Could you check a few things on this model? Use its own coordinates, in mm. Face numbers are marked on the shaded views. Round coordinates to 2 decimals unless told otherwise and drop trailing zeros. Loops run counter-clockwise (first coordinate to the right, second up) from the corner with the lowest first, then second, coordinate; pieces in that order, holes last. Notation, with made-up numbers: M 57,-13.5 L 115,-13.5 A14 ccw 115,13.5 Z; hole C 81.5,12.5 d7. An arc over 180 degrees is marked long. Answer in a Markdown table with one row per item.
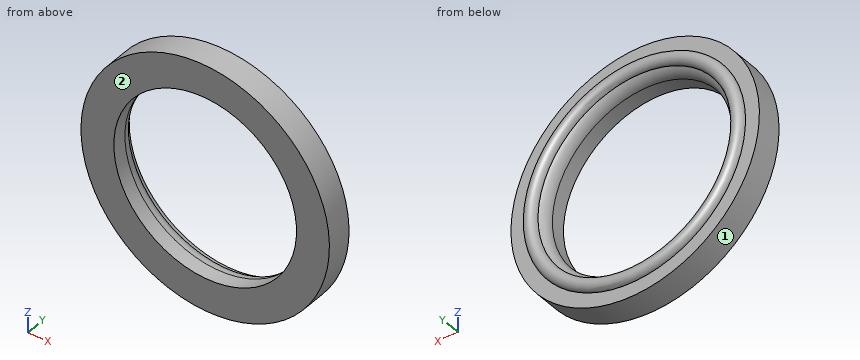
```python
from build123d import *

# Parameters (mm, degrees)
SKETCH1_R           = 23.0505
SKETCH1_R_2         = 16.9545
BOSS_EXTRUDE1_DEPTH = 4.7625
FILLET1_R           = 2.54


with BuildPart() as part:
    # Sketch1 → Boss-Extrude1 (new body)
    with BuildSketch(Plane(origin=(0, 0, 0), x_dir=(1, 0, 0), z_dir=(0, 1, 0))):
        with Locations(Location((0, 0, 0), (0, 0, 90))):
            Circle(SKETCH1_R)
        with Locations(Location((0, 0, 0), (0, 0, 90))):
            Circle(SKETCH1_R_2, mode=Mode.SUBTRACT)
    extrude(amount=BOSS_EXTRUDE1_DEPTH)

    # Sketch2 → Revolve1 (revolve)
    with BuildSketch(Plane.XY, mode=Mode.PRIVATE) as revolve1_sk:
        with BuildLine():
            Line((18.034, 4.710412046), (20.477314517, 4.739986951))
            ThreePointArc((20.477314517, 4.739986951), (19.240869806, 5.946856757), (18.034, 4.710412046))
        make_face()
    revolve(revolve1_sk.sketch.rotate(Axis((0, 0, 0), (0, 1, 0)), 90), axis=Axis((0, 0, 0), (0, 1, 0)))

    # Fillet1
    # the kernel refuses this fillet: 2.54 mm, written as the material it takes off along each edge
    with BuildSketch(Plane(origin=(0, 4.7625, 0), x_dir=(0, 0, -1), z_dir=(1, 0, 0))) as fillet1_piece_1:
        with BuildLine():
            CenterArc((19.4945, -2.078446948), FILLET1_R, 125.086398031, 54.913601969)
            Line((18.03448004, 0), (18.005279641, 0.041568939))
            ThreePointArc((18.005279641, 0.041568939), (17.49449002, 0.0508), (16.9545, 0.0508))
            Line((16.9545, 0.0508), (16.9037, 0))
            Line((16.9037, 0), (16.9037, -2.078446948))
            Line((16.9037, -2.078446948), (16.9545, -2.078446948))
        make_face()
    revolve(axis=Axis((0, 4.7625, 0), (0, 1, 0)), mode=Mode.SUBTRACT)


solid = part.part
```
1) I want a section at B-B, the plane z = 0. Please give me the cut outline in (x, y), plus the area to 3 significant figures.
Computed:
| item | result |
|---|---|
| outline | M -23.05,0 L -16.95,0 L -16.95,2.68 A2.54 ccw -18.03,4.76 A1.22 ccw -20.48,4.76 L -23.05,4.76 Z; M 16.95,0 L 23.05,0 L 23.05,4.76 L 20.48,4.76 A1.22 ccw 18.03,4.76 A2.54 ccw 16.95,2.68 Z |
| area | 61.2 mm² |
2) If we mould it in two halves opening along X, with no side actions, what happens to the marked faces 1 and 2? For each: released by +X, released by -X, zero draft, split by the parting line, or undercut.
Computed:
| item | result |
|---|---|
| face 1 | split by the parting line |
| face 2 | zero draft |
3) I want a section at C-C, the plane y = 1.95. Please give me the cut outline in (x, z), plus the area to 3 significant figures.
Computed:
| item | result |
|---|---|
| outline | C 0,0 d46.1; hole C 0,0 d33.91 |
| area | 766 mm² |
4) Will these pins go through, and if not, where does the flat tip stop? P1, Ø1.5, axis at x = 2, y = 3, coming from the +Z side; P2, Ø2, axis at x = -15.5, z = 6.5, coming from the +Y side; P3, Ø3, axis at y = 2.5, z = 4, coming from the -X side; P4, Ø23, axis at x = -9, z = -4.5, coming from the +Y side.
Computed:
| item | result |
|---|---|
| P1 | stops at z = 23.02 |
| P2 | stops at y = 4.58 |
| P3 | stops at x = -22.91 |
| P4 | stops at y = 5.95 |
5) I want a section at A-A, the plane x = 0. Please give me the cut outline in (y, z), plus the area to 3 significant figures.
Computed:
| item | result |
|---|---|
| outline | M 0,-23.05 L 4.76,-23.05 L 4.76,-20.48 A1.22 ccw 4.76,-18.03 A2.54 ccw 2.68,-16.95 L 0,-16.95 Z; M 0,16.95 L 2.68,16.95 A2.54 ccw 4.76,18.03 A1.22 ccw 4.76,20.48 L 4.76,23.05 L 0,23.05 Z |
| area | 61.2 mm² |
6) I need wall thicknesses on line 1 (X direction, y = 0.8, z = 0); line 2 (Z direction, x = 15.5, y = 2.3); line 3 (Y direction, x = -15.5, z = 15). Which ranges of each line are inside material? Lowest first, please.
Computed:
| item | result |
|---|---|
| line 1 | x = -23.05 to -16.95, 16.95 to 23.05 |
| line 2 | z = -17.06 to -6.87, 6.87 to 17.06 |
| line 3 | y = 0 to 4.76 |
